Geometry: final body of the model. Coordinates: model frame, mm. Face numbers are marked on the shaded views. A direction names the side the tool comes from. Coordinates: 2 decimals unless noted, no trailing zeros. Loops run counter-clockwise (first coordinate to the right, second up) from the corner with the lowest first, then second, coordinate; pieces in that order, holes last. Notation, with made-up numbers: (-14, -39) -> (8, -39) arc R13 cw to (8, -33) -> close; hole circle Ø4 at (-33, 1). An arc over 180 degrees is marked (long way). One line per item, written item: value. Start each with the question number.
Item 1: Ray query, probe 1 along X at (y, z) = (-8.5, 7.5); probe 2 along X at (y, z) = (0.5, 6.25). Return the intervals inside material, ascending. Write a range as from..to.
Item 2: Section query C-C on y = -1. Return loops of the section in (x, z).
Item 3: Contact query for flat-ended pins moving along their axis: pin 1 Ø2.5 at (y, z) = (10.5, 5.5) entering from -X; pin 2 Ø4.5 at (x, z) = (7.5, 4) entering from +Y; pin 3 Ø8 at (x, z) = (6, 6.5) entering from -Y. Output: stop coordinate, or through.
Item 4: Set-up query: the marked faces 4, 5, 6 and 7. Return all of +Z, -Z, +X, -X, +Y, -Y with unobstructed straight access to the full face (end or side cutting, diameter ignored); none if empty.
Item 5: Mould query, pull axis X, two halves, no side actions, for the marked faces 1, 2 and 3. Classes: +X half, -X half, draft (parallel to the pull), parting line (faces both ways), or undercut.
Item 6: Section query A-A on x = -14. Return loops of the section in (y, z), then the cut area to 3 significant figures.
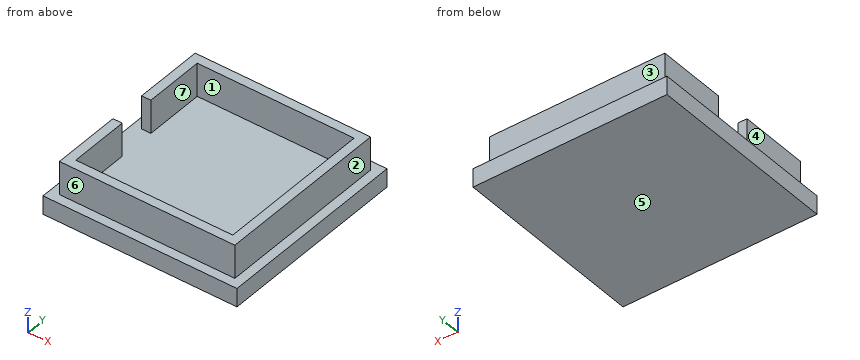
from build123d import *

# Parameters (mm, degrees)
F1_DEPTH = 9
F2_W     = 52.4
F2_H     = 52.4
F3_DEPTH = 5


with BuildPart() as f1:
    # F0 (on Top) → F1 (new body)
    with BuildSketch(Plane.XY):
        Polygon((-21.2, 21.2), (21.2, 21.2), (21.2, -21.2), (-21.2, -21.2), (-21.2, -5), (-23.7, -5), (-23.7, -23.7), (23.7, -23.7), (23.7, 23.7), (-23.7, 23.7), (-23.7, 5), (-21.2, 5), align=None)
    extrude(amount=F1_DEPTH)

    # F2 (on Top) → F3 (join)
    with BuildSketch(Plane.XY):
        Rectangle(F2_W, F2_H)
    extrude(amount=-F3_DEPTH)


solid = f1.part
Reply:
1. probe 1: x = -23.7..-21.2, 21.2..23.7
1. probe 2: x = 21.2..23.7
2. outline: (-26.2, -5) -> (26.2, -5) -> (26.2, 0) -> (23.7, 0) -> (23.7, 9) -> (21.2, 9) -> (21.2, 0) -> (-26.2, 0) -> close
3. pin 1: stops at x = -23.7
3. pin 2: stops at y = 23.7
3. pin 3: stops at y = -23.7
4. face 4: +Z, -X, +Y, -Y
4. face 5: -Z, +X, -X, +Y, -Y
4. face 6: +Z, +X, -X, -Y
4. face 7: +Z
5. face 1: undercut
5. face 2: +X half
5. face 3: draft
6. outline: (-26.2, -5) -> (26.2, -5) -> (26.2, 0) -> (23.7, 0) -> (23.7, 9) -> (21.2, 9) -> (21.2, 0) -> (-21.2, 0) -> (-21.2, 9) -> (-23.7, 9) -> (-23.7, 0) -> (-26.2, 0) -> close
6. area: 307 mm²
